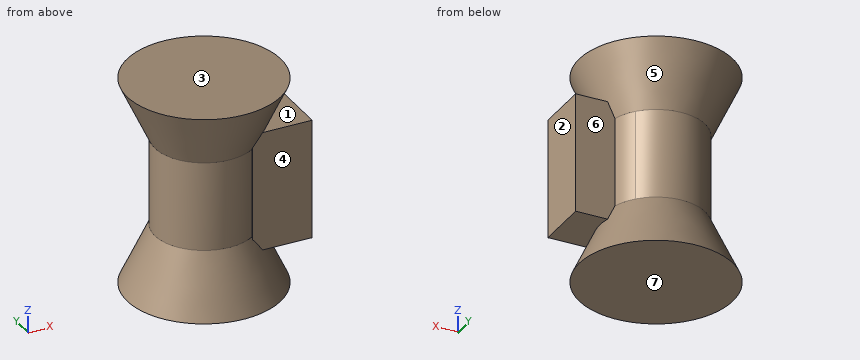
from build123d import *

# Parameters (mm, degrees)
SKETCH001_W  = 1
SKETCH001_H  = 7.5
PAD_DEPTH    = 20
SKETCH002_W  = 6
SKETCH002_H  = 12.06981
PAD001_DEPTH = 5.5


with BuildPart() as part:
    # Sketch → Revolution (revolve)
    with BuildSketch(Plane.XZ):
        Polygon((0, 0), (7.75, 0), (4.952154, 6), (4.952154, 15), (7.75, 21), (0, 21), align=None)
    revolve(axis=Axis((0, 0, 0), (0, 0, 1)))

    # Sketch001 → Pad (new body)
    with BuildSketch(Plane(origin=(0, 0, 21), x_dir=(-1, 0, 0), z_dir=(0, 0, 1))):
        with Locations((-3.25, 0.5)):
            Rectangle(SKETCH001_W, SKETCH001_H)
    extrude(amount=-PAD_DEPTH)

    # Sketch002 → Pad001 (new body)
    with BuildSketch(Plane.XZ.offset(4.25)):
        with Locations((5.75, 10.5)):
            Rectangle(SKETCH002_W, SKETCH002_H)
    extrude(amount=-PAD001_DEPTH)


solid = part.part
Read the model definition and answer for the solid it produces. Units are mm, in the model's axes. Face numbers are marked on the shaded views. A direction names the side the tool comes from. Round coordinates to 2 decimals unless told otherwise and drop trailing zeros. Write each loop counter-clockwise with the first axis right and the second up, starting at its lowest first coordinate (ties: lowest second). Pieces come first, ordered by that corner, then holes.
Q1. Flat-ended cylindrical pins translate along their axes: P1, Ø3, axis at x = 7, z = 10.5, coming from the +Y side; P2, Ø5, axis at x = 5, z = 11.5, coming from the +Y side; P3, Ø1, axis at y = -5, z = 8, coming from the -X side. Find the tip coordinate at first contact, or state that the pin passes through.
Values:
P1: stops at y = 1.25
P2: stops at y = 4.27
P3: stops at x = -2.07
Q2. Straight lines are drawn through the part: line 1 (Z direction, x = -5, y = -0.25); line 2 (Y direction, x = 5.25, z = 7.75); line 3 (X direction, y = -0.25, z = 8.5). For each, find the intervals that lie inside material, in ascending order.
Values:
line 1: z = 0 to 5.88, 15.12 to 21
line 2: y = -4.25 to 1.25
line 3: x = -4.95 to 8.75
Q3. The mould has two halves that part along Z. Classify the marked faces 1, 2 and 3: released by +Z, released by -Z, zero draft, split by the parting line, or undercut.
Values:
face 1: undercut
face 2: zero draft
face 3: released by +Z
Q4. Find section D-D on z = 18.25. Determine the outline of the cut face in (x, y).
Values:
outline: circle Ø12.94 at (0, 0)
Q5. Find section C-C on y = 0. Determine the outline of the cut face in (x, z), and give its area (3 significant figures).
Values:
outline: (-7.75, 0) - (7.75, 0) - (5.67, 4.47) - (8.75, 4.47) - (8.75, 16.53) - (5.67, 16.53) - (7.75, 21) - (-7.75, 21) - (-4.95, 15) - (-4.95, 6) - close
area: 286 mm2
Q6. A tool of negligible diameter and unlimited length cuts with its end or side. For the marked faces 4, 5, 6 and 7, from which of +Z, -Z, +X, -X, +Y, -Y can it reach the whole face along a straight path? Write none if from no direction.
Values:
face 4: +X, -Y
face 5: none
face 6: +X, +Y
face 7: -Z, +X, -X, +Y, -Y
Q7. Find section A-A on x = 0. Determine the outline of the cut face in (y, z).
Values:
outline: (-7.75, 0) - (7.75, 0) - (4.95, 6) - (4.95, 15) - (7.75, 21) - (-7.75, 21) - (-4.95, 15) - (-4.95, 6) - close
